Read the model definition and answer for the solid it produces. Units are mm, in the model's axes. Give positions to 0.01 mm unless a question says otherwise; leave off trailing zeros. Loops run counter-clockwise (first coordinate to the right, second up) from the corner with the lowest first, then second, coordinate; pieces in that order, holes last. Notation, with made-up numbers: (-40, 5) - (17, 5) arc R21 cw to (17, 31) - close; hole circle Ø4 at (51, 70). An arc over 180 degrees is marked (long way). Use a Markdown table: item, result. Add a question column.
Item 1: Consider probe 1 along Y at (x, z) = (1.8, -0.25); probe 2 along Y at (x, z) = (-1.7, 0.5); probe 3 along X at (y, z) = (1, -0.5). Determine where each line is inside the solid, lowest interval first. Write a range as [from, to].
Item 2: A cutting plane is placed at B-B (z = 2.25). Determine the outline of the cut face in (x, y), plus the area to 3 significant figures.
Item 3: A cutting plane is placed at A-A (x = 2.1). Determine the outline of the cut face in (y, z), plus the area to 3 significant figures.
Item 4: This flat-tipped pin is pushed along its axis until it touches: P1, Ø0.5, axis at x = -1.5, y = 2, coming from the -Z side. Where does it stop, or does it pass through?
from build123d import *

# Parameters (mm, degrees)
SKETCH_1_R      = 1.5
EXTRUDE_1_DEPTH = 2.35
CHAMFER_1_SIZE  = 0.3
THREAD_1_PITCH  = 0.8


with BuildPart() as part:
    # Sketch 1 → 凸台-拉伸1 (new body)
    with BuildSketch(Plane(origin=(0, 0, 0), x_dir=(1, 0, 0), z_dir=(0, 1, 0))):
        Polygon((0, 3.117691454), (-2.7, 1.558845727), (-2.7, -1.558845727), (0, -3.117691454), (2.7, -1.558845727), (2.7, 1.558845727), align=None)
        with Locations(Location((0, 0, 0), (0, 0, 270))):
            Circle(SKETCH_1_R, mode=Mode.SUBTRACT)
    extrude(amount=EXTRUDE_1_DEPTH)

    # 倒角1
    chamfer_1_edges = [part.edges().sort_by_distance(p)[0] for p in [
        (-2.7, 2.35, 0),
        (-1.35, 2.35, 2.33826859),
        (1.35, 2.35, 2.33826859),
        (2.7, 2.35, 0),
        (1.35, 2.35, -2.33826859),
        (2.7, 0, 0),
        (1.35, 0, 2.33826859),
        (-1.35, 0, 2.33826859),
        (-1.35, 2.35, -2.33826859),
        (-2.7, 0, 0),
        (-1.35, 0, -2.33826859),
        (1.35, 0, -2.33826859),
    ]]
    chamfer(chamfer_1_edges, length=CHAMFER_1_SIZE)

    # 螺纹线1: the profile of Sketch 1 2 profile screwed along a right-hand helix of 2.9375 turns, 8 arcs to a turn; built about Z, then put on its axis
    thread_1_z = Axis((0, 0, 0), (0, 0, 1))
    thread_1_corners = [(1.4997, 0, -0.000173205), (1.9330127, 0, 0.249999999), (1.9330127, 0, 0.349999999), (1.4997, 0, 0.600173203)]
    with BuildLine(mode=Mode.PRIVATE) as thread_1_profile:
        Line(thread_1_corners[0], thread_1_corners[1])
        Line(thread_1_corners[1], thread_1_corners[2])
        Line(thread_1_corners[2], thread_1_corners[3])
        Line(thread_1_corners[3], thread_1_corners[0])
    thread_1_cap = Face(thread_1_profile.wire())
    thread_1_turn_angles = [0, 22.5, 45, 67.5, 90, 112.5, 135, 157.5, 180, 202.5, 225, 247.5, 270, 292.5, 315, 337.5, 360]
    thread_1_turn_weights = [1, 0.9238795325112867, 1, 0.9238795325112867, 1, 0.9238795325112867, 1, 0.9238795325112867, 1, 0.9238795325112867, 1, 0.9238795325112867, 1, 0.9238795325112867, 1, 0.9238795325112867, 1]
    thread_1_turn_rails = [Edge.make_bspline([Vector(p[0], p[1], 0).rotate(thread_1_z, thread_1_turn_angles[k]) / thread_1_turn_weights[k] + Vector(0, 0, p[2] + THREAD_1_PITCH * thread_1_turn_angles[k] / 360) for k in range(17)], [0, 0, 0, 1, 1, 2, 2, 3, 3, 4, 4, 5, 5, 6, 6, 7, 7, 8, 8, 8], 2, thread_1_turn_weights) for p in thread_1_corners]
    thread_1_turn_sides = [Face.make_surface_from_curves(thread_1_turn_rails[p[0]], thread_1_turn_rails[p[1]]) for p in [(0, 1), (1, 2), (2, 3), (3, 0)]]
    thread_1_last_angles = [720, 742.5, 765, 787.5, 810, 832.5, 855, 877.5, 900, 922.5, 945, 967.5, 990, 1012.5, 1035, 1046.25, 1057.5]
    thread_1_last_weights = [1, 0.9238795325112867, 1, 0.9238795325112867, 1, 0.9238795325112867, 1, 0.9238795325112867, 1, 0.9238795325112867, 1, 0.9238795325112867, 1, 0.9238795325112867, 1, 0.9807852804032304, 1]
    thread_1_last_rails = [Edge.make_bspline([Vector(p[0], p[1], 0).rotate(thread_1_z, thread_1_last_angles[k]) / thread_1_last_weights[k] + Vector(0, 0, p[2] + THREAD_1_PITCH * thread_1_last_angles[k] / 360) for k in range(17)], [0, 0, 0, 1, 1, 2, 2, 3, 3, 4, 4, 5, 5, 6, 6, 7, 7, 8, 8, 8], 2, thread_1_last_weights) for p in thread_1_corners]
    thread_1_last_sides = [Face.make_surface_from_curves(thread_1_last_rails[p[0]], thread_1_last_rails[p[1]]) for p in [(0, 1), (1, 2), (2, 3), (3, 0)]]
    thread_1 = Plane(origin=(0, 2.35, 0), x_dir=(-1, 0, 0), z_dir=(0, -1, 0)) * Solid(Shell([*[p.moved(Location((0, 0, THREAD_1_PITCH * i))) for i in range(2) for p in thread_1_turn_sides], *thread_1_last_sides, thread_1_cap, thread_1_cap.rotate(thread_1_z, 1057.5).moved(Location((0, 0, THREAD_1_PITCH * 1057.5 / 360)))]))
    add(thread_1, mode=Mode.SUBTRACT)


solid = part.part
Geometry says:
| question | item | result |
|---|---|---|
| 1 | probe 1 | [0.18, 0.75], [0.98, 1.55], [1.78, 2.35] |
| 1 | probe 2 | [0, 0.34], [0.63, 1.14], [1.43, 2.35] |
| 1 | probe 3 | [-2.7, -1.58], [1.75, 2.7] |
| 2 | outline | (-1.5, 0.3) - (-0.9, 0) - (0.9, 0) - (1.5, 0.3) - (1.5, 2.05) - (0.9, 2.35) - (-0.9, 2.35) - (-1.5, 2.05) - close |
| 2 | area | 6.70 mm² |
| 3 | outline | (0, -1.56) - (0.3, -1.91) - (2.05, -1.91) - (2.35, -1.56) - (2.35, 1.56) - (2.05, 1.91) - (0.3, 1.91) - (0, 1.56) - close |
| 3 | area | 8.75 mm² |
| 4 | P1 | z = -2.4 |
